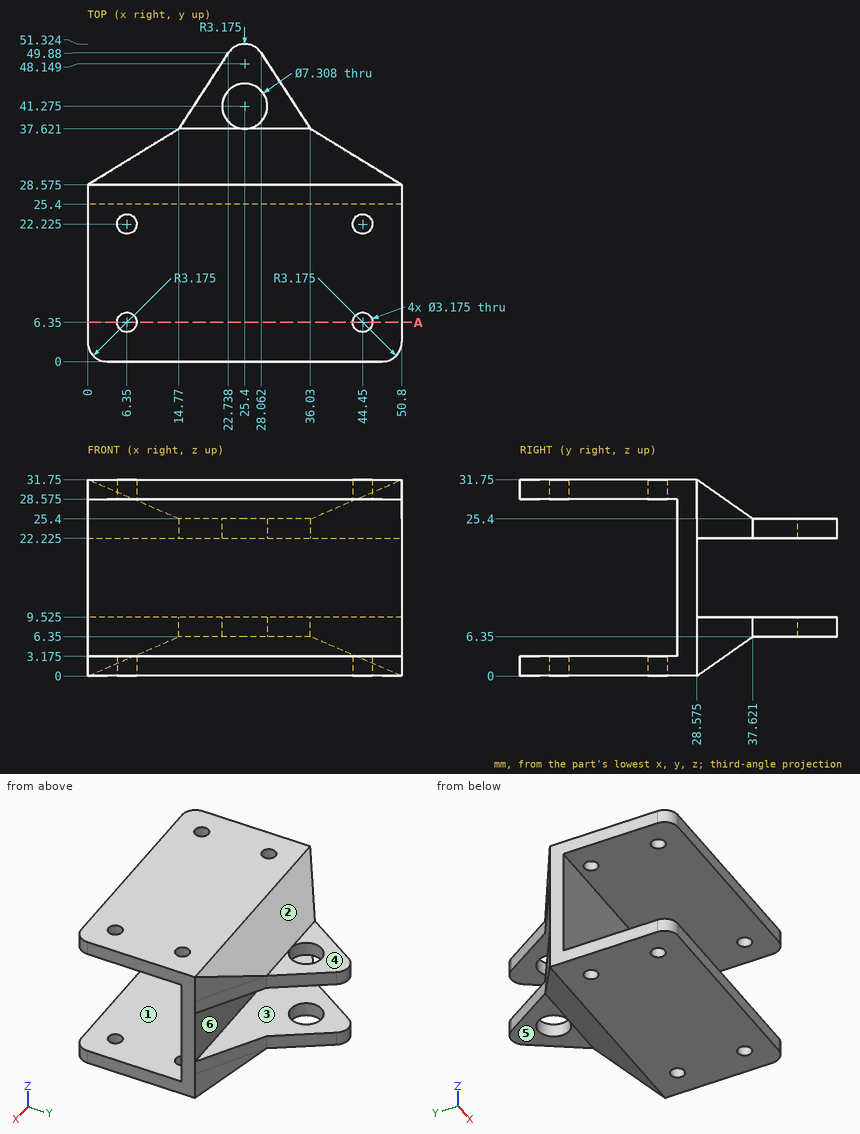
For this review, use the dimensioned drawing (mm, ordinates from the lowest corner) and the shaded views. A direction names the side the tool comes from. Give positions to 0.01 mm unless a question says otherwise; leave off trailing zeros.
Item 1: Take a section at A-A, the plane y = 6.35. Give the number of separate pieces and of enclosed holes in the cut face, and give its area (3 significant figures).
Item 2: Insertion check: pin 1 (11.5 mm diameter, centred on x = 25.4, y = 41.275, fed in from -Z); pin 2 (4 mm diameter, centred on x = 21, y = 47.5, fed in from +Z); pin 3 (7 mm diameter, centred on x = 30.5, y = 46.5, fed in from -Z). Each pin has a flat end and moves straight along its axis. Give the tip position at first contact, or say it passes through.
Item 3: Draft analysis for pull direction Z (two halves, no side actions). For the marked faces 4, 5 and 6, state which applies: +Z half, -Z half, draft (parallel to the pull), parting line (faces both ways), or undercut.
Item 4: Tool access review of the marked faces 1, 2 and 3: name each direction out of +Z, -Z, +X, -X, +Y, -Y from which nothing blocks a thin tool from reaching the whole face with its end or side.
Item 5: For line 1 along X through (y, z) = (6.35, 2); line 2 along Y through (x, z) = (25.4, 8.85) (1 decimal); line 3 along Y through (x, z) = (40, 14.5) (1 decimal), list the stretches that pass through material, from the lowest coordinate up.
Calculated:
1. separate pieces: 6
1. enclosed holes: 0
1. area: 282 mm2
2. pin 1: stops at z = 4.88
2. pin 2: stops at z = 25.4
2. pin 3: stops at z = 6.35
3. face 4: +Z half
3. face 5: -Z half
3. face 6: undercut
4. face 1: +X, -X, -Y
4. face 2: +Z, +X, -X, +Y
4. face 3: +X, -X, +Y
5. line 1: x = 0 to 4.76, 7.94 to 42.86, 46.04 to 50.8
5. line 2: y = 25.4 to 37.6, 44.9 to 51.3
5. line 3: y = 25.4 to 28.6
